The listing builds one solid part. Answer for the finished solid, in the listing's coordinates (mm). A direction names the side the tool comes from. Round coordinates to 2 decimals unless told otherwise and drop trailing zeros. Write each loop counter-clockwise with the first axis right and the second up, starting at its lowest first coordinate (ties: lowest second). Pieces come first, ordered by that corner, then holes. Notation, with made-up numbers: (27.5, 64) - (83.5, 64) arc R31 ccw to (83.5, 97) - close; hole circle Ø1 at (68.25, 47). An arc over 180 degrees is marked (long way). Answer as CSV lines item,"result". Start each with the question number.
Item 1: Which of the six approach directions +Z, -Z, +X, -X, +Y, -Y give full straight-line access (tool end or side, diameter ignored) to faces 4 (the cylindrical face through (44.1, -13.9, 12.6)), 5 (the cylindrical face through (31.31, 51.65, 9.39))?
Item 2: Straight lines are drawn through the part: line 1 along Y through (x, z) = (0, 1.75); line 2 along Y through (x, z) = (31.75, 5.5); line 3 along X through (y, z) = (54.5, 2.75). For each, find the intervals that lie inside material, in ascending order. Write a range as [from, to].
Item 3: A cutting plane is placed at B-B on y = 0. Determine the outline of the cut face in (x, z), and give its area (3 significant figures).
Item 4: For a pull along Y with two mould halves and no side action, classify faces 1 (the cylindrical face through (58.11, -30.46, 6.26)), 2 (the cylindrical face through (-60.47, 46.367, 9.392)), 3 (the flat face through (16, 35, 0)) as pulls with the +Y half, pulls with the -Y half, needs draft (parallel to the pull), parting line crosses it, or undercut.
Item 5: A cutting plane is placed at D-D on x = -63.5. Determine the outline of the cut face in (y, z), and give its area (3 significant figures).
Item 6: A cutting plane is placed at C-C on z = 1.75. State how many separate pieces and enclosed holes the cut face has, and give its area (3 significant figures).
Item 7: A cutting plane is placed at A-A on x = 0. Determine the outline of the cut face in (y, z), and give its area (3 significant figures).
Item 8: Flat-ended cylindrical pins translate along their axes: pin 1 (18 mm diameter, centred on x = 0, y = -63.5, fed in from -Z); pin 2 (5 mm diameter, centred on x = -17, z = 2, fed in from -Y); pin 3 (20 mm diameter, centred on x = -54.99, y = 31.75, fed in from +Z); pin 4 (10 mm diameter, centred on x = 50, z = 8.5, fed in from +Y). Find the tip coordinate at first contact, or state that the pin passes through.
Autodesk Inventor part; units mm, degrees
ref_plane "YZ Plane" through (0, 0, 0) normal (1, 0, 0) x (0, 1, 0)
ref_plane "XZ Plane" through (0, 0, 0) normal (0, 1, 0) x (-1, 0, 0)
ref_plane "XY Plane" through (0, 0, 0) normal (0, 0, 1) x (1, 0, 0)
sketch "Sketch1" plane through (0, 0, 0) normal (0, 0, 1) x (1, 0, 0)
  circle A0 centre (0, 0) radius 76.2
  circle A1 centre (0, 63.5) radius 3.3734
  circle A2 centre (0, 0) radius 38.1
  circle A3 centre (-31.75, 54.9926) radius 3.3734
  circle A4 centre (-54.9926, 31.75) radius 3.3734
  circle A5 centre (-63.5, 0) radius 3.3734
  circle A6 centre (-54.9926, -31.75) radius 3.3734
  circle A7 centre (-31.75, -54.9926) radius 3.3734
  circle A8 centre (0, -63.5) radius 3.3734
  circle A9 centre (31.75, -54.9926) radius 3.3734
  circle A10 centre (54.9926, -31.75) radius 3.3734
  circle A11 centre (63.5, 0) radius 3.3734
  circle A12 centre (54.9926, 31.75) radius 3.3734
  circle A13 centre (31.75, 54.9926) radius 3.3734
  dimension "d0" = 63.5
  dimension "d1" = 152.4
  dimension "d2" = 6.7469
  dimension "d3" = 76.2
  dimension "d6" = 360
extrude "Extrusion1" add sketch "Sketch1" along normal blind 6.35
sketch "Sketch2" plane through (0, 0, 6.35) normal (0, 0, 1) x (1, 0, 0)
  circle A0 centre (0, 0) radius 46.2375
  circle A1 centre (0, 0) radius 52.5875
  dimension "d10" = 92.475
  dimension "d11" = 6.35
extrude "Extrusion2" add sketch "Sketch2" along normal blind 12.7
sketch "Sketch3" plane through (0, 0, 6.35) normal (0, 0, 1) x (1, 0, 0)
  circle A0 centre (0, 63.5) radius 3.3734
  circle A1 centre (-54.9926, 31.75) radius 3.3734
  circle A2 centre (54.9926, -31.75) radius 3.3734
  circle A3 centre (0, -63.5) radius 3.3734
  circle A4 centre (-63.5, 0) radius 3.3734
  circle A5 centre (31.75, 54.9926) radius 3.3734
  circle A6 centre (-31.75, 54.9926) radius 3.3734
  circle A7 centre (54.9926, 31.75) radius 3.3734
  circle A8 centre (-31.75, -54.9926) radius 3.3734
  circle A9 centre (-54.9926, -31.75) radius 3.3734
  circle A10 centre (31.75, -54.9926) radius 3.3734
  circle A11 centre (63.5, 0) radius 3.3734
  circle A12 centre (0, 0) radius 76.2
  circle A13 centre (0, 0) radius 52.5875
extrude "Extrusion3" add sketch "Sketch3" along normal blind 12.7
sketch "Sketch4" plane through (0, 0, 19.05) normal (0, 0, 1) x (1, 0, 0)
  circle A0 centre (0, 63.5) radius 3.3734 construction
  circle A1 centre (0, 63.5) radius 11.1125
  circle A2 centre (-54.9926, 31.75) radius 11.1125
  circle A3 centre (-54.9926, -31.75) radius 11.1125
  circle A4 centre (0, -63.5) radius 11.1125
  circle A5 centre (54.9926, -31.75) radius 11.1125
  circle A6 centre (54.9926, 31.75) radius 11.1125
  point P0 (0, 0)
  dimension "d16" = 22.225
  dimension "d19" = 360
extrude "Extrusion4" cut sketch "Sketch4" against normal blind 6.35
properties part number "28521_Bearing_Holder"
Geometry says:
1,face 4,"+Z"
1,face 5,"+Z, -Z"
2,line 1,"y = [-76.2, -66.87], [-60.13, -38.1], [38.1, 60.13], [66.87, 76.2]"
2,line 2,"y = [-69.27, -58.37], [-51.62, -21.06], [21.06, 51.62], [58.37, 69.27]"
2,line 3,"x = [-53.26, -35.09], [-28.41, 28.41], [35.09, 53.26]"
3,outline,"(-76.2, 0) - (-66.87, 0) - (-66.87, 19.05) - (-76.2, 19.05) - close; (-60.13, 0) - (-38.1, 0) - (-38.1, 6.35) - (-46.24, 6.35) - (-46.24, 19.05) - (-60.13, 19.05) - close; (38.1, 0) - (60.13, 0) - (60.13, 19.05) - (46.24, 19.05) - (46.24, 6.35) - (38.1, 6.35) - close; (66.87, 0) - (76.2, 0) - (76.2, 19.05) - (66.87, 19.05) - close"
3,area,"988 mm^2"
4,face 1,"undercut"
4,face 2,"parting line crosses it"
4,face 3,"needs draft"
5,outline,"(-42.12, 0) - (-3.37, 0) - (-3.37, 19.05) - (-24.6, 19.05) - (-24.6, 12.7) - (-38.9, 12.7) - (-38.9, 19.05) - (-42.12, 19.05) - close; (3.37, 0) - (42.12, 0) - (42.12, 19.05) - (38.9, 19.05) - (38.9, 12.7) - (24.6, 12.7) - (24.6, 19.05) - (3.37, 19.05) - close"
5,area,"1,290 mm^2"
6,separate pieces,"1"
6,enclosed holes,"13"
6,area,"13,300 mm^2"
7,outline,"(-76.2, 0) - (-66.87, 0) - (-66.87, 12.7) - (-74.61, 12.7) - (-74.61, 19.05) - (-76.2, 19.05) - close; (-60.13, 0) - (-38.1, 0) - (-38.1, 6.35) - (-46.24, 6.35) - (-46.24, 19.05) - (-52.39, 19.05) - (-52.39, 12.7) - (-60.13, 12.7) - close; (38.1, 0) - (60.13, 0) - (60.13, 12.7) - (52.39, 12.7) - (52.39, 19.05) - (46.24, 19.05) - (46.24, 6.35) - (38.1, 6.35) - close; (66.87, 0) - (76.2, 0) - (76.2, 19.05) - (74.61, 19.05) - (74.61, 12.7) - (66.87, 12.7) - close"
7,area,"791 mm^2"
8,pin 1,"stops at z = 0"
8,pin 2,"stops at y = -74.81"
8,pin 3,"stops at z = 12.7"
8,pin 4,"stops at y = 61.49"
